from build123d import *

# Parameters (mm, degrees)
SKETCH_1_W          = 36
SKETCH_1_H          = 51.3
EXTRUDE_1_DEPTH     = 3
CUT_EXTRUDE_1_DEPTH = 3
SKETCH_5_W          = 30.38
SKETCH_5_H          = 30.38
SKETCH_4_W          = 35
SKETCH_4_H          = 35
FILLET_1_R          = 2
CUT_EXTRUDE_3_DEPTH = 13
FILLET_2_R          = 2
SKETCH_8_R          = 2.75
CUT_EXTRUDE_4_DEPTH = 0.5
MM_2_D              = 2
MM_2_DEPTH          = 5
MM_2_TIP            = 0.600860619
CUT_EXTRUDE_START   = 10
SKETCH_16_W         = 13
SKETCH_16_H         = 6
CUT_EXTRUDE_5_DEPTH = 9.0000001


with BuildPart() as part:
    # 草图1 → 凸台-拉伸1 (new body)
    with BuildSketch(Plane(origin=(0, 0, 0), x_dir=(1, 0, 0), z_dir=(0, 1, 0))):
        Rectangle(SKETCH_1_W, SKETCH_1_H)
    extrude(amount=EXTRUDE_1_DEPTH)

    # 草图2 → 切除-拉伸1 (cut)
    with BuildSketch(Plane(origin=(0, 3, 0), x_dir=(1, 0, 0), z_dir=(0, 1, 0))):
        with BuildLine():
            Line((-6, 23.15), (6, 23.15))
            ThreePointArc((6, 23.15), (7.75, 21.4), (6, 19.65))
            Line((6, 19.65), (-6, 19.65))
            ThreePointArc((-6, 19.65), (-7.75, 21.4), (-6, 23.15))
        make_face()
        with BuildLine():
            Line((-6, -23.15), (6, -23.15))
            ThreePointArc((6, -23.15), (7.75, -21.4), (6, -19.65))
            Line((6, -19.65), (-6, -19.65))
            ThreePointArc((-6, -19.65), (-7.75, -21.4), (-6, -23.15))
        make_face()
    extrude(amount=-CUT_EXTRUDE_1_DEPTH, mode=Mode.SUBTRACT)

    # 草图5 → 放样1 section 0
    with BuildSketch(Plane(origin=(0, 16, 0), x_dir=(1, 0, 0), z_dir=(0, 1, 0))):
        Rectangle(SKETCH_5_W, SKETCH_5_H)
    # 草图4 → 放样1 section 1
    with BuildSketch(Plane(origin=(0, 3, 0), x_dir=(1, 0, 0), z_dir=(0, 1, 0))):
        Rectangle(SKETCH_4_W, SKETCH_4_H)
    loft()

    # 圆角1
    fillet_1_edges = [part.edges().sort_by_distance(p)[0] for p in [
        (0, 16, 15.19),
        (-15.19, 16, 0),
        (0, 16, -15.19),
        (15.19, 16, 0),
        (16.345, 9.5, -16.345),
        (16.345, 9.5, 16.345),
        (-16.345, 9.5, 16.345),
        (-16.345, 9.5, -16.345),
    ]]
    fillet(fillet_1_edges, radius=FILLET_1_R)

    # 草图6 → 切除-拉伸3 (cut)
    with BuildSketch(Plane(origin=(0, 3, 0), x_dir=(1, 0, 0), z_dir=(0, 1, 0))):
        Polygon((-8.5, 25.65), (-11.75, 18), (-18, 18), (-18, 25.65), align=None)
        Polygon((18, 25.65), (8.5, 25.65), (11.75, 18), (18, 18), align=None)
        Polygon((8.5, -25.65), (11.75, -18), (18, -18), (18, -25.65), align=None)
        Polygon((-18, -25.65), (-8.5, -25.65), (-11.75, -18), (-18, -18), align=None)
    extrude(amount=-CUT_EXTRUDE_3_DEPTH, mode=Mode.SUBTRACT)

    # 圆角2
    fillet_2_edges = [part.edges().sort_by_distance(p)[0] for p in [
        (-8.5, 1.5, -25.65),
        (-11.75, 1.5, -18),
        (-18, 1.5, -18),
        (18, 1.5, -18),
        (11.75, 1.5, -18),
        (8.5, 1.5, -25.65),
        (8.5, 1.5, 25.65),
        (11.75, 1.5, 18),
        (18, 1.5, 18),
        (-18, 1.5, 18),
        (-11.75, 1.5, 18),
        (-8.5, 1.5, 25.65),
    ]]
    fillet(fillet_2_edges, radius=FILLET_2_R)

    # 草图8 → 切除-拉伸4 (cut)
    with BuildSketch(Plane.XZ):
        with Locations((-11.75, 11.75)):
            Circle(SKETCH_8_R)
        with Locations((11.75, -11.75)):
            Circle(SKETCH_8_R)
    extrude(amount=-CUT_EXTRUDE_4_DEPTH, mode=Mode.SUBTRACT)

    # 大小mm 暗销孔2
    with Locations(Plane(origin=(0, 0, 0), x_dir=(-1, 0, 0), z_dir=(0, -1, 0))):
        with Locations((11.75, -11.75), (-11.75, 11.75)):
            Hole(MM_2_D / 2, depth=MM_2_DEPTH)
            with Locations((0, 0, -(MM_2_DEPTH + MM_2_TIP / 2))):  # 118° drill point
                Cone(0, MM_2_D / 2, MM_2_TIP, mode=Mode.SUBTRACT)

    # 草图16 → 切除-拉伸5 (cut, through all)
    with BuildSketch(Plane(origin=(0, 0, 0), x_dir=(0, 0, -1), z_dir=(1, 0, 0)).offset(CUT_EXTRUDE_START)):
        with Locations((0, 6)):
            Rectangle(SKETCH_16_W, SKETCH_16_H)
    extrude(amount=CUT_EXTRUDE_5_DEPTH, mode=Mode.SUBTRACT)


solid = part.part
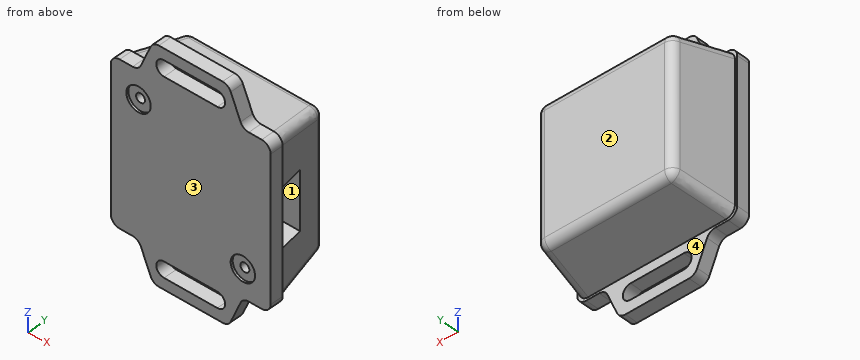
Part model, mm, in its own coordinate system. Face numbers are marked on the shaded views. A direction names the side the tool comes from. Round coordinates to 2 decimals unless told otherwise and drop trailing zeros. Order: outer loops, then holes, each group sorted by start corner. A loop starts at its lowest first (then second) coordinate and runs counter-clockwise, first axis right, second up. Notation, with made-up numbers: (13.5, 53) -> (72.5, 53) arc R17 ccw to (72.5, 81) -> close; hole circle Ø1 at (31, -19). An arc over 180 degrees is marked (long way). Put each result on its own line as item: value.
Q1. Pull direction Z, two halves, no side cores. Call the marked faces 3 and 4: pulls with the +Z half, pulls with the -Z half, needs draft (parallel to the pull), parting line crosses it, or undercut.
From the geometry:
face 3: needs draft
face 4: undercut
Q2. Tool access for the marked faces 1 and 2: list every direction of +Z, -Z, +X, -X, +Y, -Y with a clear straight run to the whole face (end or side of a thin tool).
From the geometry:
face 1: +X
face 2: +Z, -Z, +X, -X, +Y
Q3. Band-saw the part on A-A (z = 20.5). Give the cut face in (x, y), and give its area (3 significant figures).
From the geometry:
outline: (-10.69, 0) -> (-7.5, 0) -> (-7.5, 3) -> (-10.69, 3) -> close; (7.5, 0) -> (10.69, 0) -> (10.69, 3) -> (7.5, 3) -> close
area: 19.1 mm2
Q4. Band-saw the part on B-B (x = -4.5). State how many separate pieces and enclosed holes the cut face has, and give its area (3 significant figures).
From the geometry:
separate pieces: 3
enclosed holes: 0
area: 557 mm2
Q5. Wall check: line 1 (Z direction, x = 11.75, y = 3.75); line 2 (Z direction, x = 11.75, y = 0.15); line 3 (Z direction, x = -11.75, y = 3.5). Give the ranges that are in metal, low to high. Write a range as [from, to].
From the geometry:
line 1: z = [-17.37, -12.75], [-10.75, -6.5], [6.5, 17.37]
line 2: z = [-18.5, -14.5], [-9, 18.5]
line 3: z = [-17.41, 10.75], [12.75, 17.41]
Q6. Pin check, flat tips, straight feed: pin 1 Ø1.5 at (y, z) = (6.5, 8) entering from -X; pin 2 Ø1.5 at (x, y) = (14, 1) entering from -Z; pin 3 Ø2.5 at (x, y) = (15, 1.5) entering from +Z. Stop position of each tip, or through.
From the geometry:
pin 1: stops at x = -17.01
pin 2: stops at z = -18
pin 3: stops at z = 18
